from build123d import *

# Parameters (mm, degrees)
SKETCH1_W              = 304.8
SKETCH1_H              = 304.622712027
BOSS_EXTRUDE1_DEPTH    = 6.35
CUT_EXTRUDE1_START     = -6.35
CUT_EXTRUDE1_OUTLINE_R = 1.7
CUT_EXTRUDE1_OUTLINE_W = 46
CUT_EXTRUDE1_OUTLINE_H = 130.477204634
CUT_EXTRUDE1_DEPTH     = 6.35
SKETCH4_W              = 85.216118386
SKETCH4_H              = 49.623018197
CUT_EXTRUDE2_DEPTH     = 10
SKETCH5_R              = 1.7
CUT_EXTRUDE3_DEPTH     = 21
SKETCH6_R              = 1.7
CUT_EXTRUDE4_DEPTH     = 21
SKETCH7_W              = 114.3
SKETCH7_H              = 69.85
CUT_EXTRUDE5_DEPTH     = 10


# Read off the part's stored shape, not the designer's step: Cut-Extrude1
with BuildPart() as part:
    # Sketch1 → Boss-Extrude1 (new body)
    with BuildSketch(Plane.XY):
        with Locations((152.4, 152.311356014)):
            Rectangle(SKETCH1_W, SKETCH1_H)
    extrude(amount=BOSS_EXTRUDE1_DEPTH)

    # Cut-Extrude1 outline → Cut-Extrude1 (cut)
    with BuildSketch(Plane.XY.offset(6.35).offset(CUT_EXTRUDE1_START)):
        with Locations((169.9, 101.950028876)):
            Circle(CUT_EXTRUDE1_OUTLINE_R)
        with Locations((152.4, 180.037397769)):
            Rectangle(CUT_EXTRUDE1_OUTLINE_W, CUT_EXTRUDE1_OUTLINE_H)
        with Locations((125.4, 247.82572008)):
            Circle(CUT_EXTRUDE1_OUTLINE_R)
        with Locations((179.4, 247.82572008)):
            Circle(CUT_EXTRUDE1_OUTLINE_R)
        with Locations((134.9, 101.950028876)):
            Circle(CUT_EXTRUDE1_OUTLINE_R)
    extrude(amount=CUT_EXTRUDE1_DEPTH, mode=Mode.SUBTRACT)

    # Sketch4 → Cut-Extrude2 (cut)
    with BuildSketch(Plane(origin=(0, 0, 0), x_dir=(-1, 0, 0), z_dir=(0, 0, -1))):
        with Locations((-152.4, 284.018084638)):
            Rectangle(SKETCH4_W, SKETCH4_H)
    extrude(amount=-CUT_EXTRUDE2_DEPTH, mode=Mode.SUBTRACT)

    # Sketch5 → Cut-Extrude3 (cut)
    with BuildSketch(Plane.XY.offset(6.35)):
        with Locations((241.35, 299.711356013)):
            Circle(SKETCH5_R)
        with Locations((266.35, 299.711356013)):
            Circle(SKETCH5_R)
        with Locations((38.45, 299.711356013)):
            Circle(SKETCH5_R)
        with Locations((63.45, 299.711356013)):
            Circle(SKETCH5_R)
        with Locations((241.35, 19.000000001)):
            Circle(SKETCH5_R)
        with Locations((241.35, 6.000000001)):
            Circle(SKETCH5_R)
        with Locations((266.35, 19.000000001)):
            Circle(SKETCH5_R)
        with Locations((266.35, 6.000000001)):
            Circle(SKETCH5_R)
        with Locations((63.45, 6)):
            Circle(SKETCH5_R)
        with Locations((38.45, 6)):
            Circle(SKETCH5_R)
        with Locations((63.45, 19)):
            Circle(SKETCH5_R)
        with Locations((38.45, 19)):
            Circle(SKETCH5_R)
    extrude(amount=-CUT_EXTRUDE3_DEPTH, mode=Mode.SUBTRACT)

    # Sketch6 → Cut-Extrude4 (cut)
    with BuildSketch(Plane.XY.offset(6.35)):
        with Locations((289.349981069, 299.740865879)):
            Circle(SKETCH6_R)
        with Locations((15.45, 299.711356012)):
            Circle(SKETCH6_R)
    extrude(amount=-CUT_EXTRUDE4_DEPTH, mode=Mode.SUBTRACT)

    # Sketch7 → Cut-Extrude5 (cut)
    with BuildSketch(Plane.XY.offset(6.35)):
        Polygon((0, 253.822712027), (0, 50.8), (69.85, 120.65), (69.85, 183.972712027), align=None)
        with Locations((152.4, 34.925)):
            Rectangle(SKETCH7_W, SKETCH7_H)
        Polygon((234.95, 120.65), (304.8, 50.8), (304.8, 253.822712027), (234.95, 183.972712027), align=None)
    extrude(amount=-CUT_EXTRUDE5_DEPTH, mode=Mode.SUBTRACT)


solid = part.part
Verification items for the finished model (mm, model axes). A direction names the side the tool comes from. Round coordinates to 2 decimals unless told otherwise and drop trailing zeros. Loops run counter-clockwise (first coordinate to the right, second up) from the corner with the lowest first, then second, coordinate; pieces in that order, holes last. Notation, with made-up numbers: M 51.25,30.5 L 96.25,30.5 A19 ccw 96.25,63.5 Z; hole C 18.25,-18.75 d10. An arc over 180 degrees is marked long. Write each question's results on one line, items separated by ' | '.
1) Gauge pin test, flat ends, axial feed: P1, Ø2, axis at x = 147.5, y = 113.5, coming from the -Z side; P2, Ø1.5, axis at y = 75, z = 3.5, coming from the +X side; P3, Ø3, axis at x = 129, z = 4.5, coming from the -Y side; P4, Ø2, axis at x = 176.5, z = 2.5, coming from the +Y side. Record the tip position at first contact, or that the pin passes through.
Checks:
P1: stops at z = 0 | P2: stops at x = 281.35 | P3: stops at y = 69.85 | P4: stops at y = 259.21
2) Section check B-B on x = 23. Record the boundary of the cut face in (y, z), then the cut area to 3 significant figures.
Checks:
outline: M 0,0 L 73.8,0 L 73.8,6.35 L 0,6.35 Z; M 230.82,0 L 304.62,0 L 304.62,6.35 L 230.82,6.35 Z | area: 937 mm2
3) Section check D-D on z = 2. State how many separate pieces and enclosed holes the cut face has, then the cut area to 3 significant figures.
Checks:
separate pieces: 1 | enclosed holes: 19 | area: 56,200 mm2
4) Mould release check, pull along Y, two halves, no side actions. Record for faces 1 (the flat face through (35.41, 218.41, 3.22)), 2 (the flat face through (270.364, 219.387, 3.219)), 3 (the flat face through (116, 154, 6.35)): released by +Y, released by -Y, zero draft, split by the parting line, or undercut.
Checks:
face 1: undercut | face 2: undercut | face 3: zero draft
5) Section check C-C on x = 186. Record the boundary of the cut face in (y, z).
Checks:
outline: M 69.85,0 L 259.21,0 L 259.21,6.35 L 69.85,6.35 Z
6) Scan lines: L1, parallel to Y at x = 169.9, z = 4; L2, parallel to Y at x = 137.5, z = 1.5; L3, parallel to X at y = 28, z = 6. Record each from-to range of solid material in increasing order. Write a range as from..to.
Checks:
L1: y = 69.85..100.25, 103.65..114.8, 245.28..259.21 | L2: y = 69.85..114.8, 245.28..259.21 | L3: x = 0..95.25, 209.55..304.8
7) Access from +Z, -Z, +X, -X, +Y, -Y to the whole of each face (thin tool, end or side, straight path). Record for faces 4 (the flat face through (34.4, 85.2, 3.2)), 5 (the flat face through (184, 154, 0)), 6 (the flat face through (269.4, 86.2, 3.2)).
Checks:
face 4: +Z, -Z, -X | face 5: -Z, +X, -X, +Y, -Y | face 6: +Z, -Z, +X
8) Section check A-A on y = 63. Record the boundary of the cut face in (x, z).
Checks:
outline: M 12.2,0 L 95.25,0 L 95.25,6.35 L 12.2,6.35 Z; M 209.55,0 L 292.6,0 L 292.6,6.35 L 209.55,6.35 Z
